Could you check a few things on this model? Use its own coordinates, in mm. A direction names the side the tool comes from. Coordinates: 2 decimals unless noted, no trailing zeros. Loops run counter-clockwise (first coordinate to the right, second up) from the corner with the lowest first, then second, coordinate; pieces in that order, holes last. Notation, with made-up numbers: (58, -35.75) -> (104, -35.75) arc R24 cw to (104, -1.75) -> close; hole circle Ø6 at (41, 50.5). An arc over 180 degrees is marked (long way). One line per question, with ' | ' between items.
```python
from build123d import *

# Parameters (mm, degrees)
SKETCH1_W           = 300
SKETCH1_H           = 200
BOSS_EXTRUDE1_DEPTH = 50
FILLET1_R           = 10
SHELL1_T            = -3


with BuildPart() as part:
    # Sketch1 → Boss-Extrude1 (new body)
    with BuildSketch(Plane(origin=(0, 0, 0), x_dir=(1, 0, 0), z_dir=(0, 1, 0))):
        Rectangle(SKETCH1_W, SKETCH1_H)
    extrude(amount=BOSS_EXTRUDE1_DEPTH)

    # Fillet1
    fillet1_edges = [part.edges().sort_by_distance(p)[0] for p in [
        (0, 0, -100),
        (150, 0, 0),
        (0, 0, 100),
        (-150, 0, 0),
        (-150, 25, -100),
        (150, 25, -100),
        (150, 25, 100),
        (-150, 25, 100),
    ]]
    fillet(fillet1_edges, radius=FILLET1_R)

    # Shell1
    shell1_openings = [part.faces().sort_by_distance(p)[0] for p in [
        (0, 50, 0),
    ]]
    offset(amount=SHELL1_T, openings=shell1_openings, kind=Kind.INTERSECTION)


solid = part.part
```
Q1. Imagine slicing it at B-B on y = 31. Write out the boundary of the cut face in (x, z), plus the area to 3 significant figures.
Values follow:
outline: (-150, -90) arc R10 ccw to (-140, -100) -> (140, -100) arc R10 ccw to (150, -90) -> (150, 90) arc R10 ccw to (140, 100) -> (-140, 100) arc R10 ccw to (-150, 90) -> close; hole (-147, -90) arc R7 ccw to (-140, -97) -> (140, -97) arc R7 ccw to (147, -90) -> (147, 90) arc R7 ccw to (140, 97) -> (-140, 97) arc R7 ccw to (-147, 90) -> close | area: 2,920 mm2
Q2. We'd pull the mould along X, two halves only. Please class faces 3 (the face through (-147.15, 30.28, -96.99)), 4 (the face through (146.99, 30.28, 97.15)), 5 (the face through (-145, 30.3, 94.9)): released by +X, released by -X, zero draft, split by the parting line, or undercut.
Values follow:
face 3: released by -X | face 4: released by +X | face 5: undercut
Q3. Imagine slicing it at A-A on x = 87. Write out the boundary of the cut face in (y, z).
Values follow:
outline: (0, -90) arc R10 ccw to (10, -100) -> (50, -100) -> (50, -97) -> (10, -97) arc R7 cw to (3, -90) -> (3, 90) arc R7 cw to (10, 97) -> (50, 97) -> (50, 100) -> (10, 100) arc R10 ccw to (0, 90) -> close
Q4. For pin 1 (2 mm diameter, centred on y = 5, z = 66.5, fed in from +X); pin 2 (8 mm diameter, centred on x = 54.5, z = 60, fed in from +Y); pin 3 (8 mm diameter, centred on x = 116.5, y = 7.5, fed in from -Z), each with a flat end and sliding along its axis, tell me the tip position at first contact or that it passes through.
Values follow:
pin 1: stops at x = 149.17 | pin 2: stops at y = 3 | pin 3: stops at z = -100
Q5. Please list where these lines run through material, in increasing order: L1, parallel to Z at x = -132.5, y = 23.5; L2, parallel to X at y = 17.5, z = -48; L3, parallel to X at y = 8.5, z = 60. Write a range as [from, to].
Values follow:
L1: z = [-100, -97], [97, 100] | L2: x = [-150, -147], [147, 150] | L3: x = [-149.89, -146.84], [146.84, 149.89]
Q6. For faces 1 (the face through (147, 30, 1)), 2 (the face through (-2, 0, -1)), which set-ups out of +Z, -Z, +X, -X, +Y, -Y let a thin tool reach every point of the face, with its end or its side?
Values follow:
face 1: +Y | face 2: +Z, -Z, +X, -X, -Y
Q7. Imagine slicing it at C-C on z = 41.5. Write out the boundary of the cut face in (x, y), plus the area to 3 significant figures.
Values follow:
outline: (-150, 10) arc R10 ccw to (-140, 0) -> (140, 0) arc R10 ccw to (150, 10) -> (150, 50) -> (147, 50) -> (147, 10) arc R7 cw to (140, 3) -> (-140, 3) arc R7 cw to (-147, 10) -> (-147, 50) -> (-150, 50) -> close | area: 1,160 mm2
